Input: part model. Units: mm. Frame: model coordinates. A direction names the side the tool comes from. Give positions to 0.01 mm unless a question says otherwise; leave off trailing zeros. Order: outer loops, then holes, each group sorted by start corner. A loop starts at its lowest first (then second) coordinate and runs counter-clockwise, first axis right, second up. Notation, with made-up numbers: (-11, 46.5) - (5, 46.5) arc R27 ccw to (5, 82.5) - close; hole circle Ø8 at (79.5, 41). An arc over 180 degrees is marked (long way). Answer in a Markdown table with one row per item. Add a question column.
from build123d import *

# Parameters (mm, degrees)
SKETCH1_W           = 17.38
SKETCH1_H           = 47.498
BOSS_EXTRUDE1_DEPTH = 5.95
CUT_EXTRUDE1_DEPTH  = 3.41
SKETCH3_W           = 10.16
SKETCH3_H           = 2.54
BOSS_EXTRUDE2_DEPTH = 7.62


with BuildPart() as part:
    # Sketch1 → Boss-Extrude1 (new body)
    with BuildSketch(Plane.XY):
        Rectangle(SKETCH1_W, SKETCH1_H)
    extrude(amount=BOSS_EXTRUDE1_DEPTH)

    # Sketch2 → Cut-Extrude1 (cut)
    with BuildSketch(Plane.XY.offset(5.95)):
        with BuildLine():
            Line((-6.189150765, -7.510055771), (-4.375543678, -7.510055771))
            add(Edge.make_bspline(
                [(-4.375543678, -7.510055771), (-4.236100034, -7.508741028), (-3.965259686, -7.506187413), (-3.575157739, -7.462880983), (-3.212929647, -7.401011341), (-2.879952148, -7.312618696), (-2.576880198, -7.195940416), (-2.299787614, -7.059475133), (-2.057227298, -6.889398664), (-1.839886176, -6.696896273), (-1.6506173, -6.473748397), (-1.49147229, -6.216884478), (-1.351582714, -5.931396028), (-1.240365711, -5.611742151), (-1.156767721, -5.260026908), (-1.093019054, -4.878648158), (-1.055622823, -4.465737579), (-1.052313767, -4.18021236), (-1.050597351, -4.03210967)],
                knots=[0, 0, 0, 0, 1.200271823, 2.331279013, 3.375715191, 4.363218718, 5.292340221, 6.169095557, 7.016022317, 7.835399336, 8.663899785, 9.525803296, 10.431341886, 11.396986964, 12.433702812, 13.541488193, 14.724763392, 16, 16, 16, 16], degree=3))
            Line((-1.050597351, -4.03210967), (-1.050597351, 3.823122672))
            add(Edge.make_bspline(
                [(-1.050597351, 3.823122672), (-1.050990706, 4.018476815), (-1.051722861, 4.38209167), (-1.082819341, 4.883729691), (-1.123621868, 5.300544302), (-1.186312233, 5.642512462), (-1.277849339, 5.934194205), (-1.409859259, 6.190898998), (-1.576026296, 6.428387627), (-1.712615445, 6.564129267), (-1.782010909, 6.633094146)],
                knots=[0, 0, 0, 0, 1.563811524, 2.910739897, 4.022716534, 4.915381324, 5.690198038, 6.460778295, 7.217983238, 8, 8, 8, 8], degree=3))
            add(Edge.make_bspline(
                [(-1.782010909, 6.633094146), (-1.857869082, 6.699334544), (-2.010689546, 6.832779473), (-2.266570655, 7.006932331), (-2.552722511, 7.147733735), (-2.863765744, 7.261431627), (-3.198352588, 7.358338614), (-3.560509802, 7.416582757), (-3.947751905, 7.461850273), (-4.214926271, 7.464099814), (-4.353153467, 7.465263653)],
                knots=[0, 0, 0, 0, 0.872288361, 1.757272915, 2.673228345, 3.628310148, 4.624832827, 5.686398416, 6.803018934, 8, 8, 8, 8], degree=3))
            Line((-4.353153467, 7.465263653), (-5.700297825, 7.465263653))
            Line((-5.700297825, 7.465263653), (-5.700297825, 7.90933617))
            add(Edge.make_bspline(
                [(-5.700297825, 7.90933617), (-5.451430477, 7.922958599), (-4.966965958, 7.949477079), (-4.25899913, 8.010023738), (-3.589407964, 8.083563347), (-2.954434187, 8.172799954), (-2.352988403, 8.280285748), (-1.78214455, 8.408269267), (-1.238010952, 8.547978741), (-0.715430392, 8.715533332), (-0.195727602, 8.910375221), (0.33741676, 9.132306906), (0.886154119, 9.39705879), (1.256038344, 9.587742493), (1.44591117, 9.685626239)],
                knots=[0, 0, 0, 0, 1.206551741, 2.348767378, 3.4393851, 4.467302093, 5.452435193, 6.396265705, 7.29893257, 8.171177332, 9.051491902, 9.98535699, 10.965822455, 12, 12, 12, 12], degree=3))
            Line((1.44591117, 9.685626239), (2.293007484, 9.685626239))
            Line((2.293007484, 9.685626239), (2.293007484, -4.457523678))
            add(Edge.make_bspline(
                [(2.293007484, -4.457523678), (2.294317311, -4.580815267), (2.296865591, -4.820680062), (2.340584624, -5.167266406), (2.402324898, -5.491083353), (2.490852806, -5.790612798), (2.608465987, -6.064671603), (2.745851868, -6.318652921), (2.914467795, -6.54690087), (3.110897203, -6.749009464), (3.329168057, -6.930218955), (3.572808862, -7.08810542), (3.844565821, -7.217801947), (4.140194362, -7.32714774), (4.462230563, -7.407047666), (4.808870425, -7.466843235), (5.180494619, -7.504994367), (5.437493331, -7.508338715), (5.569441686, -7.510055771)],
                knots=[0, 0, 0, 0, 1.151629664, 2.240504938, 3.259800832, 4.230940235, 5.153094675, 6.043018888, 6.924394745, 7.796053501, 8.671426729, 9.571246426, 10.502083077, 11.480572872, 12.512719618, 13.598486478, 14.767014217, 16, 16, 16, 16], degree=3))
            Line((5.569441686, -7.510055771), (7.244975806, -7.510055771))
            Line((7.244975806, -7.510055771), (7.244975806, -7.987713605))
            Line((7.244975806, -7.987713605), (-6.189150765, -7.987713605))
            Line((-6.189150765, -7.987713605), (-6.189150765, -7.510055771))
        make_face()
    extrude(amount=-CUT_EXTRUDE1_DEPTH, mode=Mode.SUBTRACT)

    # Sketch3 → Boss-Extrude2 (add)
    with BuildSketch(Plane(origin=(0, 23.749, 0), x_dir=(1, 0, 0), z_dir=(0, 1, 0))):
        with Locations((0, -2.975)):
            Rectangle(SKETCH3_W, SKETCH3_H)
    extrude(amount=BOSS_EXTRUDE2_DEPTH)


solid = part.part
Q1. Section B-B, the plane y = -2. Return loops of the section in (x, z), then the cut area to 3 significant figures.
Q2. Section A-A, the plane x = 6.75. Return loops of the section in (y, z), then the cut area to 3 significant figures.
Q3. Pull-direction query (Y, two-part tool) for faces 6 (the flat face through (6, -7.51, 4)), 7 (the flat face through (0, 28, 4.245)), 8 (the flat face through (2.293, 3, 4)), 9 (the flat face through (0, -23.749, 3)); classes: +Y half, -Y half, draft (parallel to the pull), parting line (faces both ways), or undercut.
Q4. Access query for faces 1 (the flat face through (0, 28, 1.705)), 2 (the flat face through (1, 0, 2.54)), 3 (the flat face through (5.08, 28, 3)), 4 (the flat face through (8.69, 0, 3)), 5 (the flat face through (-5.08, 28, 3)). Directions: +Z, -Z, +X, -X, +Y, -Y. A direction counts if a zero-diameter tool reaches every point of the face in a straight line with its end or side. Return the directions, or none.
Q5. Line query: probe 1 along Y at (x, z) = (-6, 3); probe 2 along Y at (x, z) = (-4.75, 4.1); probe 3 along Y at (x, z) = (4.25, 5.45). Output: solid intervals per line, ascending.
Q6. Contact query for a flat-ended pin moving along its axis: P1, Ø2, axis at y = 27, z = 3, coming from the +X side. Output: stop coordinate, or through.
Q7. Section C-C, the plane z = 0.55. Return loops of the section in (x, y), then the cut area to 3 significant figures.
Computed:
| question | item | result |
|---|---|---|
| 1 | outline | (-8.69, 0) - (8.69, 0) - (8.69, 5.95) - (2.29, 5.95) - (2.29, 2.54) - (-1.05, 2.54) - (-1.05, 5.95) - (-8.69, 5.95) - close |
| 1 | area | 92.0 mm^2 |
| 2 | outline | (-23.75, 0) - (23.75, 0) - (23.75, 5.95) - (-7.51, 5.95) - (-7.51, 2.54) - (-7.99, 2.54) - (-7.99, 5.95) - (-23.75, 5.95) - close |
| 2 | area | 281 mm^2 |
| 3 | face 6 | undercut |
| 3 | face 7 | draft |
| 3 | face 8 | undercut |
| 3 | face 9 | -Y half |
| 4 | face 1 | -Z, +X, -X, +Y |
| 4 | face 2 | +Z |
| 4 | face 3 | +Z, -Z, +X, +Y |
| 4 | face 4 | +Z, -Z, +X, +Y, -Y |
| 4 | face 5 | +Z, -Z, -X, +Y |
| 5 | probe 1 | y = -23.75 to -7.99, -7.51 to 23.75 |
| 5 | probe 2 | y = -23.75 to -7.99, -7.51 to 7.47, 7.97 to 31.37 |
| 5 | probe 3 | y = -23.75 to -7.99, -7.35 to 23.75 |
| 6 | P1 | stops at x = 5.08 |
| 7 | outline | (-8.69, -23.75) - (8.69, -23.75) - (8.69, 23.75) - (-8.69, 23.75) - close |
| 7 | area | 826 mm^2 |
